Here's the drawing with two shaded views (mm, measured from the low corner). I have some questions. A direction names the side the tool comes from. Round coordinates to 2 decimals unless told otherwise and drop trailing zeros. Write each loop counter-clockwise with the first axis right and the second up, starting at its lowest first coordinate (ties: lowest second). Pieces come first, ordered by that corner, then holes. Notation, with made-up numbers: M 59,87.25 L 72,87.25 A8 ccw 72,91.25 Z; hole C 48,60 d6. An arc over 180 degrees is marked long. Write item = value, one per line. Start each with the question number.
(1) Will these pins go through, and if not, where does the flat tip stop? pin 1 Ø4 at (y, z) = (20, 6) entering from +X; pin 2 Ø0.9 at (x, y) = (13.5, 9) entering from +Z; pin 3 Ø5 at (y, z) = (9, 7.5) entering from +X.
(2) I want a section at B-B (z = 6). List the corners of the cut face in (x, y) for me, and give its area (3 significant figures).
(3) I want a section at A-A (y = 11.25). List the corners of the cut face in (x, z) for me, and give its area (3 significant figures).
(4) If we mould it in two halves opening along X, with no side actions, what happens to the marked faces 4, 5 and 6? For each: released by +X, released by -X, zero draft, split by the parting line, or undercut.
(5) I need wall thicknesses on line 1 along Y through (x, z) = (13.75, 10.8); line 2 along Z through (x, y) = (20.75, 8); line 3 along Y through (x, z) = (11, 7). Which ranges of each line are inside material? Lowest first, please.
(6) On a 3-axis mill with a long thin cutter (end or side, diameter ignored), from which of +Z, -Z, +X, -X, +Y, -Y can I reach the whole of each face in a straight line? I mean the marked faces 1, 2 and 3. Say none if no direction works.
(7) I want a section at C-C (x = 11.25). List the corners of the cut face in (y, z) for me.
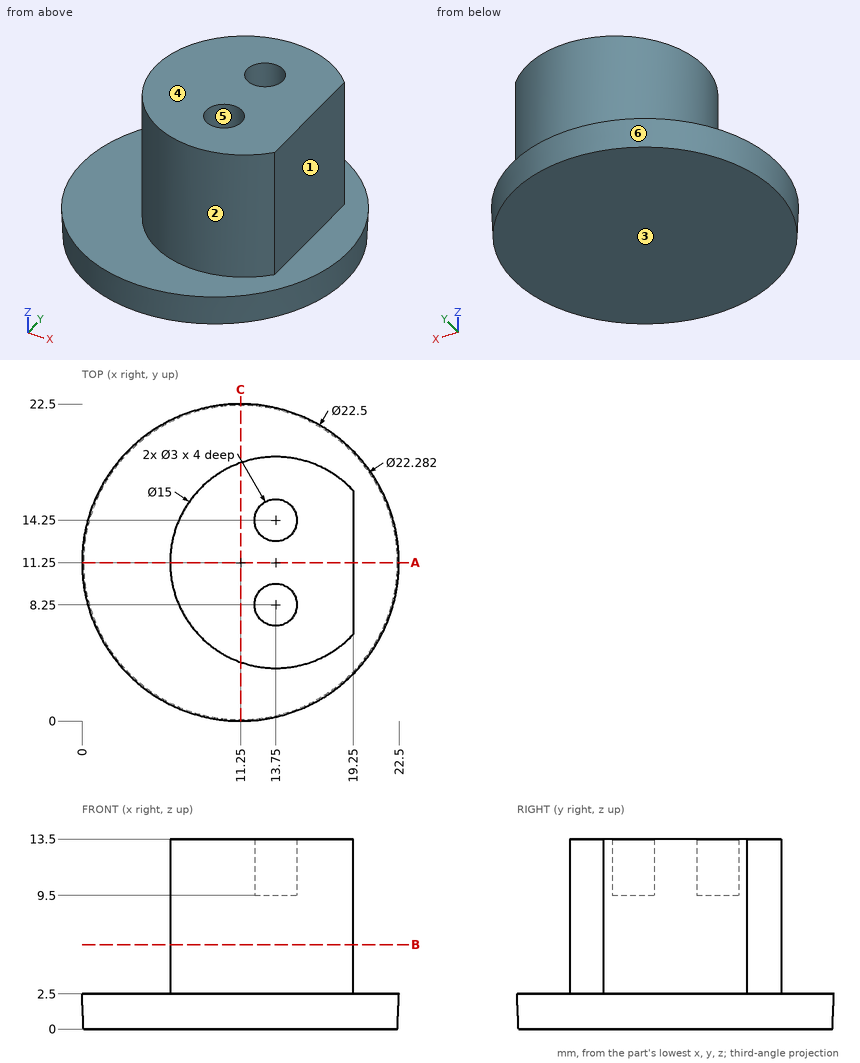
Returned:
q1.pin_1 = 17.02
q1.pin_2 = 9.5
q1.pin_3 = 19.25
q2.outline = M 19.25,6.15 L 19.25,16.35 A7.5 ccw long Z
q2.area = 163 mm²
q3.outline = M 0,2.5 L 0.11,0 L 22.39,0 L 22.5,2.5 L 19.25,2.5 L 19.25,13.5 L 6.25,13.5 L 6.25,2.5 Z
q3.area = 199 mm²
q4.face_4 = zero draft
q4.face_5 = undercut
q4.face_6 = split by the parting line
q5.line_1 = 3.75 to 6.75, 9.75 to 12.75, 15.75 to 18.75
q5.line_2 = 0 to 2.5
q5.line_3 = 4.27 to 18.23
q6.face_1 = +Z, +X, +Y, -Y
q6.face_2 = +Z
q6.face_3 = -Z, +X, -X, +Y, -Y
q7.outline = M 0,2.5 L 0.11,0 L 22.39,0 L 22.5,2.5 L 18.32,2.5 L 18.32,13.5 L 4.18,13.5 L 4.18,2.5 Z
